Could you check a few things on this model? Use its own coordinates, in mm. A direction names the side the tool comes from. Coordinates: 2 decimals unless noted, no trailing zeros. Order: outer loops, then holes, each group sorted by start corner. A loop starts at its lowest first (then second) coordinate and runs counter-clockwise, first axis right, second up. Notation, with made-up numbers: (70.25, 77.5) - (94.25, 77.5) arc R32 cw to (94.25, 111.5) - close; hole circle Ø5 at (84, 43.5). An arc over 180 degrees is marked (long way). Answer as a JSON object with one key per item and string values. Group by question number.
(1) Will these pins go through, and if not, where does the flat tip stop? P1, Ø5.5, axis at x = -116.31, y = 95, coming from the -Z side; P2, Ø1.5, axis at y = 42.5, z = 1, coming from the -X side; P3, Ø1.5, axis at y = 82, z = 2.5, coming from the +X side; P4, Ø1.5, axis at x = -68.5, z = 2, coming from the +Y side.
(2) Imagine slicing it at B-B, the plane y = 95. Write out the boundary of the cut face in (x, z).
(3) Imagine slicing it at C-C, the plane x = -7. Write out the boundary of the cut face in (y, z).
(4) Imagine slicing it at A-A, the plane y = 26. Write out the boundary of the cut face in (x, z).
(5) Which directions (+Z, -Z, +X, -X, +Y, -Y) give clear straight access to the entire face, cutting with the end or side of a thin tool? Please do faces 5 (the flat face through (-82, 43, 1)), 6 (the cylindrical face through (-2, 1, 2)).
(6) We'd pull the mould along X, two halves only. Please class faces 1 (the cylindrical face through (-78.99, 2.85, 1.52)), 2 (the cylindrical face through (-7.338, 28.578, 1.479)), 3 (the flat face through (-69, 44, 3)), 4 (the cylindrical face through (-0.871, 30.285, 1.521)): pulls with the +X half, pulls with the -X half, needs draft (parallel to the pull), parting line crosses it, or undercut.
(7) Please list where these lines run through material, in increasing order: probe 1 along X at (y, z) = (64, 2.65); probe 2 along Y at (x, z) = (-7, 1.95); probe 3 along X at (y, z) = (92.5, 1.9).
(8) Imagine slicing it at D-D, the plane z = 0.75. Write out the boundary of the cut face in (x, y), and give its area (3 significant figures).
from build123d import *

# Parameters (mm, degrees)
ESBO_O1_R                = 2.6
RESSALTO_EXTRUS_O1_DEPTH = 3
FILETE2_R                = 110
FILETE3_R                = 4
RESSALTO_EXTRUS_O2_DEPTH = 3
FILETE4_R                = 10
FILETE5_R                = 10
FILETE6_R                = 5
ESBO_O3_R                = 3.05
CORTE_EXTRUS_O1_DEPTH    = 10


with BuildPart() as part:
    # Esboço1 → Ressalto-extrusão1 (new body)
    with BuildSketch(Plane.XY):
        with BuildLine():
            Line((-82, 75), (-82, 0))
            Line((-82, 0), (0, 0))
            Line((0, 0), (0, 31))
            Line((0, 31), (-62, 31))
            Line((-62, 31), (-62, 75))
            ThreePointArc((-62, 75), (-99.43321729, 111.660780356), (-135.305624889, 73.47139772))
            Line((-135.305624889, 73.47139772), (-135.305624889, 63.47139772))
            Line((-135.305624889, 63.47139772), (-115.3375, 75))
            ThreePointArc((-115.3375, 75), (-98.66875, 91.66875), (-82, 75))
        make_face()
        with Locations((-7, 26)):
            Circle(ESBO_O1_R, mode=Mode.SUBTRACT)
        with Locations((-73.8, 15)):
            Circle(ESBO_O1_R, mode=Mode.SUBTRACT)
        with Locations((-7, 4)):
            Circle(ESBO_O1_R, mode=Mode.SUBTRACT)
    extrude(amount=RESSALTO_EXTRUS_O1_DEPTH)

    # Filete2
    # the kernel refuses this fillet: 110 mm, written as the material it adds along each edge
    with BuildSketch(Plane(origin=(-62, 31, 0), x_dir=(1, 0, 0), z_dir=(0, 0, 1))) as filete2_piece_1_section:
        with BuildLine():
            CenterArc((97.045462199, 104.267998826), FILETE2_R, 204.262159278, 47.159856314)
            Line((-3.238772458, 59.067641757), (-13.267195924, 54.54760605))
            ThreePointArc((-13.267195924, 54.54760605), (-11, 44), (-11, 0))
            Line((-11, 0), (0, -11))
            ThreePointArc((0, -11), (31, -11), (58.49545378, -10.426799883))
            Line((58.49545378, -10.426799883), (62, 0))
        make_face()
    filete2_piece_1 = extrude(amount=3, mode=Mode.PRIVATE)
    filete2_piece_1 = filete2_piece_1 - Plane(origin=(-7, 26, 1.5), x_dir=(1, 0, 0), z_dir=(0, 0, -1)) * Cylinder(2.6, 255, mode=Mode.PRIVATE)
    add(filete2_piece_1)

    # Filete3
    filete3_edges = [part.edges().sort_by_distance(p)[0] for p in [
        (-135.305624889, 63.47139772, 1.5),
    ]]
    fillet(filete3_edges, radius=FILETE3_R)

    # Esboço2 → Ressalto-extrusão2 (add, through all)
    with BuildSketch(Plane.XY.offset(3)):
        with BuildLine():
            ThreePointArc((-129.305624889, 66.935499335), (-133.305624889, 66.935499335), (-135.305624889, 70.39960095))
            Line((-135.305624889, 70.39960095), (-135.305624889, 55))
            Line((-135.305624889, 55), (-115.3375, 55))
            Line((-115.3375, 55), (-115.3375, 75))
            Line((-115.3375, 75), (-129.305624889, 66.935499335))
        make_face()
    extrude(amount=-RESSALTO_EXTRUS_O2_DEPTH)

    # Filete4
    # the kernel refuses this fillet: 10 mm, written as the material it takes off along each edge
    with BuildSketch(Plane(origin=(-135.305624889, 55, 28), x_dir=(0, 1, 0), z_dir=(0, 0, -1)), Plane(origin=(-115.3375, 55, 28), x_dir=(-1, 0, 0), z_dir=(0, 0, -1))) as filete4_piece_1:
        with BuildLine():
            CenterArc((FILETE4_R, FILETE4_R), FILETE4_R, 180, 90)
            Line((0, FILETE4_R), (0, 0))
            Line((0, 0), (FILETE4_R, 0))
        make_face()
    extrude(amount=53, mode=Mode.SUBTRACT)

    # Filete5
    filete5_edges = [part.edges().sort_by_distance(p)[0] for p in [
        (-82, 0, 1.5),
    ]]
    fillet(filete5_edges, radius=FILETE5_R)

    # Filete6
    filete6_edges = [part.edges().sort_by_distance(p)[0] for p in [
        (0, 31, 1.5),
        (0, 0, 1.5),
    ]]
    fillet(filete6_edges, radius=FILETE6_R)

    # Esboço3 → Corte-extrusão1 (cut)
    with BuildSketch(Plane.XY.offset(3)):
        with Locations((-125.3375, 65)):
            Circle(ESBO_O3_R)
        with Locations((-116.31024162, 95)):
            Circle(ESBO_O3_R)
        with Locations((-81.02725838, 95)):
            Circle(ESBO_O3_R)
    extrude(amount=-CORTE_EXTRUS_O1_DEPTH, mode=Mode.SUBTRACT)


solid = part.part
Result set:
{
 "1": {"P1": "passes through", "P2": "stops at x = -82", "P3": "stops at x = -60.78", "P4": "stops at y = 96.89"},
 "2": {"outline": "(-129.4, 0) - (-119.36, 0) - (-119.36, 3) - (-129.4, 3) - close; (-113.26, 0) - (-84.08, 0) - (-84.08, 3) - (-113.26, 3) - close; (-77.98, 0) - (-67.93, 0) - (-67.93, 3) - (-77.98, 3) - close"},
 "3": {"outline": "(0, 0) - (1.4, 0) - (1.4, 3) - (0, 3) - close; (6.6, 0) - (23.4, 0) - (23.4, 3) - (6.6, 3) - close; (28.6, 0) - (33.62, 0) - (33.62, 3) - (28.6, 3) - close"},
 "4": {"outline": "(-82, 0) - (-9.6, 0) - (-9.6, 3) - (-82, 3) - close; (-4.4, 0) - (0, 0) - (0, 3) - (-4.4, 3) - close"},
 "5": {"face 5": "+Z, -Z, -Y", "face 6": "+Z, -Z, +X, -Y"},
 "6": {"face 1": "pulls with the -X half", "face 2": "undercut", "face 3": "needs draft", "face 4": "pulls with the +X half"},
 "7": {"probe 1": "x = -135.26 to -128.22, -122.46 to -115.39, -82 to -48.75", "probe 2": "y = 0 to 1.4, 6.6 to 23.4, 28.6 to 33.62", "probe 3": "x = -130.89 to -118.06, -114.56 to -82.77, -79.28 to -66.45"},
 "8": {"outline": "(-135.31, 65) arc R10 ccw to (-125.32, 55) arc R10 ccw to (-115.34, 65) - (-115.34, 75) arc R16.67 cw to (-82, 75) - (-82, 10) arc R10 ccw to (-72, 0) - (-5, 0) arc R5 ccw to (0, 5) - (0, 27.47) arc R5 ccw to (-3.26, 32.15) arc R110 cw to (-65.24, 90.07) arc R36.67 ccw to (-135.31, 73.47) - close; hole circle Ø6.1 at (-125.34, 65); hole circle Ø6.1 at (-116.31, 95); hole circle Ø6.1 at (-81.03, 95); hole circle Ø5.2 at (-73.8, 15); hole circle Ø5.2 at (-7, 4); hole circle Ø5.2 at (-7, 26)", "area": "6,480 mm^2"}
}
